Verification items for the finished model (mm, model axes). A direction names the side the tool comes from. Round coordinates to 2 decimals unless told otherwise and drop trailing zeros. Order: outer loops, then holes, each group sorted by start corner. A loop starts at its lowest first (then second) coordinate and runs counter-clockwise, first axis right, second up. Notation, with made-up numbers: M -5.5,57 L 20.5,57 A28 ccw 20.5,81 Z; hole C 56.25,39 d10. An arc over 180 degrees is marked long. Use CSV: the item, a comma, the result in double quotes. Start each with the question number.
Q1. Sectioned sample at B-B (z = 25). Enter the section's corners in (x, y).
Q2. Scan lines: line 1 (Z direction, x = -3, y = -47.5); line 2 (Z direction, x = -0.75, y = 88); line 3 (Y direction, x = 2.25, z = -27.5). Record each from-to range of solid material in increasing order.
Q3. Set-up check for faces 1 (the face through (0, 53, 18)), 2 (the face through (-3.05, -2, 1)): record each of +Z, -Z, +X, -X, +Y, -Y from which the full face is reachable in a straight line by a thin tool's end or side.
Q4. Sectioned sample at C-C (y = -9). Enter the section's corners in (x, z).
Q5. Sectioned sample at D-D (x = -1). State how many separate pieces and enclosed holes the cut face has, and give its area (3 significant figures).
Q6. Mould release check, pull along Y, two halves, no side actions. Record for faces 3 (the face through (3.05, -2, -1)), 4 (the face through (0, -96, 32)): +Y half, -Y half, draft (parallel to the pull), parting line (faces both ways), or undercut.
Q7. Sectioned sample at A-A (y = 43). Enter the section's corners in (x, z).
```python
from build123d import *

# Parameters (mm, degrees)
F1_DEPTH = 110
F3_DEPTH = 6.1
F4_W     = 220
F4_H     = 15.7
F5_DEPTH = 100


with BuildPart() as f1:
    # F0 (on Front) → F1 (new body, symmetric)
    with BuildSketch(Plane.XZ):
        with BuildLine():
            ThreePointArc((11.95, -69.2), (5.6567496474, -66.5932503526), (3.05, -60.3))
            Line((3.05, -60.3), (3.05, 60.3))
            ThreePointArc((3.05, 60.3), (5.6567496474, 66.5932503526), (11.95, 69.2))
            Line((11.95, 69.2), (76, 69.2))
            Line((76, 69.2), (76, 76))
            Line((76, 76), (-76, 76))
            Line((-76, 76), (-76, 69.2))
            Line((-76, 69.2), (-11.95, 69.2))
            ThreePointArc((-11.95, 69.2), (-5.6567496474, 66.5932503526), (-3.05, 60.3))
            Line((-3.05, 60.3), (-3.05, -60.3))
            ThreePointArc((-3.05, -60.3), (-5.6567496474, -66.5932503526), (-11.95, -69.2))
            Line((-11.95, -69.2), (-76, -69.2))
            Line((-76, -69.2), (-76, -76))
            Line((-76, -76), (76, -76))
            Line((76, -76), (76, -69.2))
            Line((76, -69.2), (11.95, -69.2))
        make_face()
    extrude(amount=F1_DEPTH, both=True)

    # F2 (on face) → F3 (cut)
    with BuildSketch(Plane.YZ.offset(3.05)):
        with BuildLine():
            Line((-20.2647186258, -9), (-2.5, -9))
            Line((-2.5, -9), (-2.5, 9))
            Line((-2.5, 9), (-20.2647186258, 9))
            ThreePointArc((-20.2647186258, 9), (-24.0595842402, 6.0501256289), (-28.75, 5))
            Line((-28.75, 5), (-78.75, 5))
            ThreePointArc((-78.75, 5), (-83.4404157598, 6.0501256289), (-87.2352813742, 9))
            Line((-87.2352813742, 9), (-105, 9))
            Line((-105, 9), (-105, -9))
            Line((-105, -9), (-87.2352813742, -9))
            ThreePointArc((-87.2352813742, -9), (-83.4404157598, -6.0501256289), (-78.75, -5))
            Line((-78.75, -5), (-28.75, -5))
            ThreePointArc((-28.75, -5), (-24.0595842402, -6.0501256289), (-20.2647186258, -9))
        make_face()
        with BuildLine():
            ThreePointArc((-20.2647186258, 32), (-24.0595842402, 29.0501256289), (-28.75, 28))
            Line((-28.75, 28), (-78.75, 28))
            ThreePointArc((-78.75, 28), (-83.4404157598, 29.0501256289), (-87.2352813742, 32))
            Line((-87.2352813742, 32), (-105, 32))
            Line((-105, 32), (-105, 14))
            Line((-105, 14), (-87.2352813742, 14))
            ThreePointArc((-87.2352813742, 14), (-83.4404157598, 16.9498743711), (-78.75, 18))
            Line((-78.75, 18), (-28.75, 18))
            ThreePointArc((-28.75, 18), (-24.0595842402, 16.9498743711), (-20.2647186258, 14))
            Line((-20.2647186258, 14), (-2.5, 14))
            Line((-2.5, 14), (-2.5, 32))
            Line((-2.5, 32), (-20.2647186258, 32))
        make_face()
        with BuildLine():
            ThreePointArc((-28.75, -28), (-24.0595842402, -29.0501256289), (-20.2647186258, -32))
            Line((-20.2647186258, -32), (-2.5, -32))
            Line((-2.5, -32), (-2.5, -14))
            Line((-2.5, -14), (-20.2647186258, -14))
            ThreePointArc((-20.2647186258, -14), (-24.0595842402, -16.9498743711), (-28.75, -18))
            Line((-28.75, -18), (-78.75, -18))
            ThreePointArc((-78.75, -18), (-83.4404157598, -16.9498743711), (-87.2352813742, -14))
            Line((-87.2352813742, -14), (-105, -14))
            Line((-105, -14), (-105, -32))
            Line((-105, -32), (-87.2352813742, -32))
            ThreePointArc((-87.2352813742, -32), (-83.4404157598, -29.0501256289), (-78.75, -28))
            Line((-78.75, -28), (-28.75, -28))
        make_face()
        with BuildLine():
            Line((78.75, 28), (28.75, 28))
            ThreePointArc((28.75, 28), (24.0595842402, 29.0501256289), (20.2647186258, 32))
            Line((20.2647186258, 32), (2.5, 32))
            Line((2.5, 32), (2.5, 14))
            Line((2.5, 14), (20.2647186258, 14))
            ThreePointArc((20.2647186258, 14), (24.0595842402, 16.9498743711), (28.75, 18))
            Line((28.75, 18), (78.75, 18))
            ThreePointArc((78.75, 18), (83.4404157598, 16.9498743711), (87.2352813742, 14))
            Line((87.2352813742, 14), (105, 14))
            Line((105, 14), (105, 32))
            Line((105, 32), (87.2352813742, 32))
            ThreePointArc((87.2352813742, 32), (83.4404157598, 29.0501256289), (78.75, 28))
        make_face()
        with BuildLine():
            ThreePointArc((20.2647186258, -32), (24.0595842402, -29.0501256289), (28.75, -28))
            Line((28.75, -28), (78.75, -28))
            ThreePointArc((78.75, -28), (83.4404157598, -29.0501256289), (87.2352813742, -32))
            Line((87.2352813742, -32), (105, -32))
            Line((105, -32), (105, -14))
            Line((105, -14), (87.2352813742, -14))
            ThreePointArc((87.2352813742, -14), (83.4404157598, -16.9498743711), (78.75, -18))
            Line((78.75, -18), (28.75, -18))
            ThreePointArc((28.75, -18), (24.0595842402, -16.9498743711), (20.2647186258, -14))
            Line((20.2647186258, -14), (2.5, -14))
            Line((2.5, -14), (2.5, -32))
            Line((2.5, -32), (20.2647186258, -32))
        make_face()
        with BuildLine():
            ThreePointArc((20.2647186258, -9), (24.0595842402, -6.0501256289), (28.75, -5))
            Line((28.75, -5), (78.75, -5))
            ThreePointArc((78.75, -5), (83.4404157598, -6.0501256289), (87.2352813742, -9))
            Line((87.2352813742, -9), (105, -9))
            Line((105, -9), (105, 9))
            Line((105, 9), (87.2352813742, 9))
            ThreePointArc((87.2352813742, 9), (83.4404157598, 6.0501256289), (78.75, 5))
            Line((78.75, 5), (28.75, 5))
            ThreePointArc((28.75, 5), (24.0595842402, 6.0501256289), (20.2647186258, 9))
            Line((20.2647186258, 9), (2.5, 9))
            Line((2.5, 9), (2.5, -9))
            Line((2.5, -9), (20.2647186258, -9))
        make_face()
    extrude(amount=-F3_DEPTH, mode=Mode.SUBTRACT)

    # F4 (on face) → F5 (cut, symmetric)
    with BuildSketch(Plane.YZ.offset(3.05)):
        with Locations((0, 68.15)):
            Rectangle(F4_W, F4_H)
        with Locations((0, -68.15)):
            Rectangle(F4_W, F4_H)
    extrude(amount=F5_DEPTH, both=True, mode=Mode.SUBTRACT)


solid = f1.part
```
Verdict:
1,outline,"M -3.05,-110 L 3.05,-110 L 3.05,-105 L -3.05,-105 Z; M -3.05,-2.5 L 3.05,-2.5 L 3.05,2.5 L -3.05,2.5 Z; M -3.05,105 L 3.05,105 L 3.05,110 L -3.05,110 Z"
2,line 1,"z = -60.3 to -28, -18 to -5, 5 to 18, 28 to 60.3"
2,line 2,"z = -60.3 to -32, -14 to -9, 9 to 14, 32 to 60.3"
2,line 3,"y = -110 to -105, -2.5 to 2.5, 105 to 110"
3,face 1,"+X, -X"
3,face 2,"+Z, -Z, -X, +Y, -Y"
4,outline,"M -3.05,-60.3 L 3.05,-60.3 L 3.05,-32 L -3.05,-32 Z; M -3.05,-14 L 3.05,-14 L 3.05,-9 L -3.05,-9 Z; M -3.05,9 L 3.05,9 L 3.05,14 L -3.05,14 Z; M -3.05,32 L 3.05,32 L 3.05,60.3 L -3.05,60.3 Z"
5,separate pieces,"1"
5,enclosed holes,"6"
5,area,"18,400 mm²"
6,face 3,"draft"
6,face 4,"undercut"
7,outline,"M -3.05,-60.3 L 3.05,-60.3 L 3.05,-28 L -3.05,-28 Z; M -3.05,-18 L 3.05,-18 L 3.05,-5 L -3.05,-5 Z; M -3.05,5 L 3.05,5 L 3.05,18 L -3.05,18 Z; M -3.05,28 L 3.05,28 L 3.05,60.3 L -3.05,60.3 Z"
